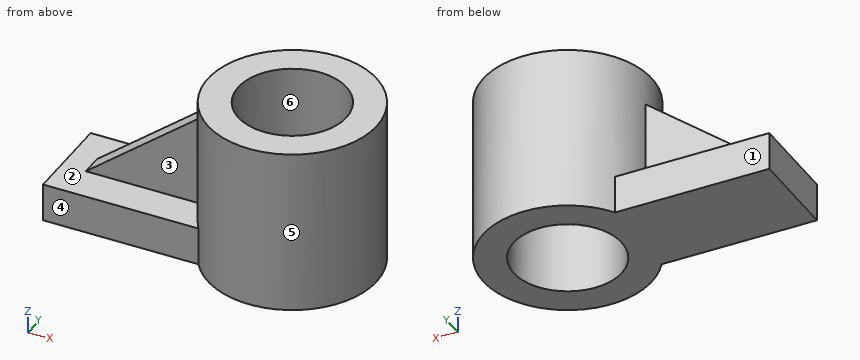
from build123d import *

# Parameters (mm, degrees)
F0_R     = 35.316834
F0_R_2   = 22.645268
F1_DEPTH = 69.596
F3_DEPTH = 16.002
F4_W     = 31.616599
F4_H     = 9.21494
F5_DEPTH = 55.372
F6_W     = 26.249159
F6_H     = 9.21494
F7_DEPTH = 39.37
F9_DEPTH = 38.1


with BuildPart() as f1:
    # F0 (on Top) → F1 (new body)
    with BuildSketch(Plane.XY):
        with Locations((35.493162, 0)):
            Circle(F0_R)
        with Locations((35.493162, 0)):
            Circle(F0_R_2, mode=Mode.SUBTRACT)
    extrude(amount=F1_DEPTH)

    # F2 (on face) → F3 (join)
    with BuildSketch(Plane(origin=(0, 0, 0), x_dir=(1, 0, 0), z_dir=(0, 0, -1))):
        with BuildLine():
            Line((-58.806233, -19.13999), (5.812536, -19.13999))
            ThreePointArc((5.812536, -19.13999), (0.178957, 0.430922), (6.288416, 19.858539))
            Line((6.288416, 19.858539), (-58.806233, 19.858539))
            Line((-58.806233, 19.858539), (-58.806233, -19.13999))
        make_face()
    extrude(amount=-F3_DEPTH)

    # F4 (on face) → F5 (join)
    with BuildSketch(Plane(origin=(0, 0, 0), x_dir=(1, 0, 0), z_dir=(0, 0, -1))):
        with Locations((-6.637758, 0)):
            Rectangle(F4_W, F4_H)
    extrude(amount=-F5_DEPTH)

    # F6 (on face) → F7 (join)
    with BuildSketch(Plane.XY.offset(16.002)):
        with Locations((-35.570636, 0)):
            Rectangle(F6_W, F6_H)
    extrude(amount=F7_DEPTH)

    # F8 (on face) → F9 (cut)
    with BuildSketch(Plane.XZ.offset(4.60747)):
        Polygon((-48.695216, 16.002), (0.478165, 55.372), (-48.695216, 55.372), align=None)
    extrude(amount=-F9_DEPTH, mode=Mode.SUBTRACT)


solid = f1.part
Part model, mm, in its own coordinate system. Face numbers are marked on the shaded views. A direction names the side the tool comes from. Coordinates: 2 decimals unless noted, no trailing zeros. Write each loop counter-clockwise with the first axis right and the second up, starting at its lowest first coordinate (ties: lowest second). Pieces come first, ordered by that corner, then holes. Notation, with made-up numbers: M 36,29 L 57,29 A7 cw 57,34 Z; hole C 72,-24 d11. An arc over 180 degrees is marked long. Return JSON: item names as keys, results as strings.
1. Saw through at B-B, the plane z = 12. Write the cut outline in (x, y), then the cut area to 3 significant figures.
Determined:
{"outline": "M -58.81,-19.86 L 6.29,-19.86 A35.32 ccw long 5.81,19.14 L -58.81,19.14 Z; hole C 35.49,0 d45.29", "area": "4,680 mm²"}
2. Saw through at D-D, the plane x = -24.5. Write the cut outline in (y, z).
Determined:
{"outline": "M -19.86,0 L 19.14,0 L 19.14,16 L 4.61,16 L 4.61,35.37 L -4.61,35.37 L -4.61,16 L -19.86,16 Z"}
3. Pull direction X, two halves, no side cores. Call the marked faces 4, 5 and 6: pulls with the +X half, pulls with the -X half, needs draft (parallel to the pull), parting line crosses it, or undercut.
Determined:
{"face 4": "needs draft", "face 5": "parting line crosses it", "face 6": "undercut"}
4. Saw through at C-C, the plane x = 47. Write the cut outline in (y, z), then the cut area to 3 significant figures.
Determined:
{"outline": "M -33.39,0 L -19.5,0 L -19.5,69.6 L -33.39,69.6 Z; M 19.5,0 L 33.39,0 L 33.39,69.6 L 19.5,69.6 Z", "area": "1,930 mm²"}
5. 3-axis set-ups, long thin cutter, end or side, ignore diameter. For the marked faces 1, 2 and 3: which of +Z, -Z, +X, -X, +Y, -Y reach the whole face in a straight line?
Determined:
{"face 1": "+Z, -Z, -X, +Y", "face 2": "+Z, -X", "face 3": "+Z, -X, -Y"}
6. Probe L1, parallel to Y at x = 16, z = 40.5; L2, parallel to Y at x = -5, z = 32; L3, parallel to X at y = -13, z = 38. List the from-to ranges inside material, lowest first.
Determined:
{"L1": "-29.45 to -11.52, 11.52 to 29.45", "L2": "-4.61 to 4.61", "L3": "2.66 to 16.95, 54.04 to 68.33"}
7. Flat gauge pins, fed straight in: pin 1 Ø8 at (x, z) = (44.5, 49.5) entering from +Y; pin 2 Ø8 at (x, z) = (-26, 11.5) entering from +Y; pin 3 Ø10 at (x, z) = (-9, 49) entering from +Y; pin 4 Ø10 at (x, y) = (-38, 22.5) entering from -Z. Where does each tip first touch, or does it go through?
Determined:
{"pin 1": "y = 34.96", "pin 2": "y = 19.14", "pin 3": "y = 4.61", "pin 4": "z = 0"}
8. Saw through at A-A, the plane y = 0. Write the cut outline in (x, z).
Determined:
{"outline": "M -58.81,0 L 12.85,0 L 12.85,69.6 L 0.18,69.6 L 0.18,55.37 L 0.48,55.37 L -48.7,16 L -58.81,16 Z; M 58.14,0 L 70.81,0 L 70.81,69.6 L 58.14,69.6 Z"}
